```python
from build123d import *

# Parameters (mm, degrees)
F0_W     = 63.008573
F0_H     = 13.715997
F0_W_2   = 105.548358
F0_H_2   = 63.5
F1_DEPTH = 25.4


with BuildPart() as f1:
    # F0 (on Front) → F1 (new body)
    with BuildSketch(Plane.XZ):
        Polygon((-94.402148, 63.5), (-94.402148, 0), (-75.095862, 0), (-56.045862, 0), (-11.852148, 0), (-11.852148, 63.5), align=None)
        with Locations((-43.591575, 41.780356)):
            Rectangle(F0_W, F0_H, mode=Mode.SUBTRACT)
        with Locations((40.922031, 31.75)):
            Rectangle(F0_W_2, F0_H_2)
    extrude(amount=F1_DEPTH)


solid = f1.part
```
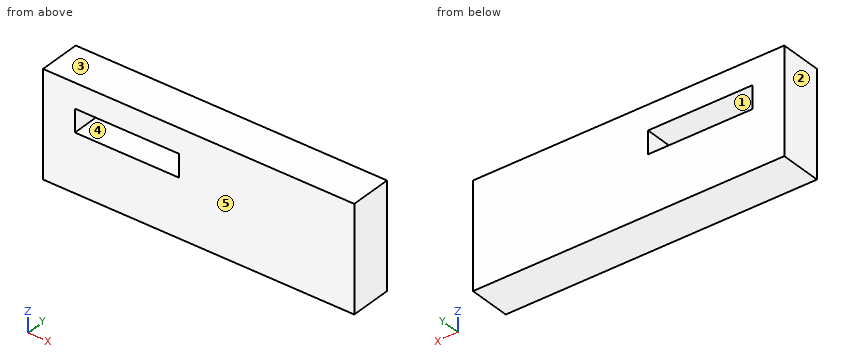
Model file for the job. Use its own axes, mm. Face numbers are marked on the shaded views. A direction names the side the tool comes from. Give positions to 0.01 mm unless a question says otherwise; leave off trailing zeros. Write each loop counter-clockwise with the first axis right and the second up, starting at its lowest first coordinate (ties: lowest second). Pieces come first, ordered by that corner, then holes. Notation, with made-up numbers: (-17, 78) -> (-9, 78) arc R19 ccw to (-9, 100) -> close; hole circle Ø6 at (39, 45). An arc over 180 degrees is marked (long way). Use CSV: the item, a comma, the result in double quotes. Start each with the question number.
1) Pin check, flat tip, straight feed: P1, Ø6, axis at x = 11, y = -16.5, coming from the -Z side. Stop position of the tip, or through.
2) Tool access for the marked faces 4 and 5: list every direction of +Z, -Z, +X, -X, +Y, -Y with a clear straight run to the whole face (end or side of a thin tool).
3) Cut at A-A on y = -5.75. List the corners of the cut face in (x, z).
4) Two-plate mould, pull along Z, no slides. Class the marked faces 1, 2 and 3: released by +Z, released by -Z, zero draft, split by the parting line, or undercut.
5) Drill centre lines: L1, parallel to Z at x = -24, y = -21; L2, parallel to X at y = -2.5, z = 47. Where is each one in solid material? Low to high.
6) Cut at B-B on x = -25. List the corners of the cut face in (y, z), plus the area to 3 significant figures.
Final values:
1,P1,"stops at z = 0"
2,face 4,"+Y, -Y"
2,face 5,"+Z, -Z, +X, -X, -Y"
3,outline,"(-94.4, 0) -> (93.7, 0) -> (93.7, 63.5) -> (-94.4, 63.5) -> close; hole (-75.1, 34.92) -> (-12.09, 34.92) -> (-12.09, 48.64) -> (-75.1, 48.64) -> close"
4,face 1,"undercut"
4,face 2,"zero draft"
4,face 3,"released by +Z"
5,L1,"z = 0 to 34.92, 48.64 to 63.5"
5,L2,"x = -94.4 to -75.1, -12.09 to 93.7"
6,outline,"(-25.4, 0) -> (0, 0) -> (0, 34.92) -> (-25.4, 34.92) -> close; (-25.4, 48.64) -> (0, 48.64) -> (0, 63.5) -> (-25.4, 63.5) -> close"
6,area,"1,260 mm2"
